Part model, mm, in its own coordinate system. A direction names the side the tool comes from. Give positions to 0.01 mm unless a question says otherwise; leave off trailing zeros. Write each loop counter-clockwise with the first axis right and the second up, starting at its lowest first coordinate (ties: lowest second). Pieces come first, ordered by that corner, then holes. Notation, with made-up numbers: M -24.5,31 L 3.5,31 A17 cw 3.5,58 Z; hole C 11,60.25 d4. An arc over 180 degrees is marked long. Answer as CSV lines item,"result". Start each with the question number.
1) Slice it at A-A, the plane y = 0. Give the cut face in (x, z), plus the area to 3 significant figures.
2) Slice it at C-C, the plane y = 7. Give the cut face in (x, z).
3) Slice it at D-D, the plane x = 5.25. Give the cut face in (y, z).
4) Tool access for faces 1 (the cylindrical face through (-3, 0, 1)), 2 (the cylindrical face through (0, -6, 1)), 3 (the cylindrical face through (-1.08, -4.88, 3.99)): list every direction of +Z, -Z, +X, -X, +Y, -Y with a clear straight run to the whole face (end or side of a thin tool).
5) Mould opens along Y. For faces 4 (the cylindrical face through (-5.95, 4.99, 1.48)), 5 (the flat face through (-1.2, 1.2, 5)), 6 (the cylindrical face through (-2.17, -9.76, 1.48)) say: pulls with the +Y half, pulls with the -Y half, needs draft (parallel to the pull), parting line crosses it, or undercut.
6) Wall check: line 1 along Y through (x, z) = (0, 2.4); line 2 along Y through (x, z) = (0, 4.25); line 3 along Z through (x, y) = (7.75, 3). Give the ranges that are in metal, low to high. Write a range as from..to.
7) Pin check, flat tips, straight feed: pin 1 Ø1.5 at (x, z) = (-1.5, 4) entering from +Y; pin 2 Ø2.5 at (x, y) = (4.95, 4.95) entering from +Z; pin 3 Ø1.8 at (x, y) = (-0.5, -0.5) entering from -Z. Stop position of each tip, or through.
```python
from build123d import *

# Parameters (mm, degrees)
SKETCH_1_R      = 10
SKETCH_1_R_2    = 3
SKETCH_1_R_3    = 1
EXTRUDE_1_DEPTH = 3
SKETCH_2_R      = 5
SKETCH_2_R_2    = 1.5
EXTRUDE_2_DEPTH = 2


with BuildPart() as part:
    # 草图1 → 凸台-拉伸1 (new body)
    with BuildSketch(Plane.XY):
        Circle(SKETCH_1_R)
        Circle(SKETCH_1_R_2, mode=Mode.SUBTRACT)
        with Locations((7, 0)):
            Circle(SKETCH_1_R_3, mode=Mode.SUBTRACT)
        with Locations((4.949747468, -4.949747468)):
            Circle(SKETCH_1_R_3, mode=Mode.SUBTRACT)
        with Locations((0, -7)):
            Circle(SKETCH_1_R_3, mode=Mode.SUBTRACT)
        with Locations((-4.949747468, -4.949747468)):
            Circle(SKETCH_1_R_3, mode=Mode.SUBTRACT)
        with Locations((-7, 0)):
            Circle(SKETCH_1_R_3, mode=Mode.SUBTRACT)
        with Locations((-4.949747468, 4.949747468)):
            Circle(SKETCH_1_R_3, mode=Mode.SUBTRACT)
        with Locations((0, 7)):
            Circle(SKETCH_1_R_3, mode=Mode.SUBTRACT)
        with Locations((4.949747468, 4.949747468)):
            Circle(SKETCH_1_R_3, mode=Mode.SUBTRACT)
    extrude(amount=EXTRUDE_1_DEPTH)

    # 草图2 → 凸台-拉伸2 (add)
    with BuildSketch(Plane.XY.offset(3)):
        Circle(SKETCH_2_R)
        Circle(SKETCH_2_R_2, mode=Mode.SUBTRACT)
    extrude(amount=EXTRUDE_2_DEPTH)


solid = part.part
```
Found:
1,outline,"M -10,0 L -8,0 L -8,3 L -10,3 Z; M -6,0 L -3,0 L -3,3 L -1.5,3 L -1.5,5 L -5,5 L -5,3 L -6,3 Z; M 1.5,3 L 3,3 L 3,0 L 6,0 L 6,3 L 5,3 L 5,5 L 1.5,5 Z; M 8,0 L 10,0 L 10,3 L 8,3 Z"
1,area,"44.0 mm²"
2,outline,"M -7.14,0 L -1,0 L -1,3 L -7.14,3 Z; M 1,0 L 7.14,0 L 7.14,3 L 1,3 Z"
3,outline,"M -8.51,0 L -5.9,0 L -5.9,3 L -8.51,3 Z; M -4,0 L 4,0 L 4,3 L -4,3 Z; M 5.9,0 L 8.51,0 L 8.51,3 L 5.9,3 Z"
4,face 1,"-Z"
4,face 2,"+Z, -Z"
4,face 3,"+Z"
5,face 4,"undercut"
5,face 5,"needs draft"
5,face 6,"parting line crosses it"
6,line 1,"-10..-8, -6..-3, 3..6, 8..10"
6,line 2,"-5..-1.5, 1.5..5"
6,line 3,"0..3"
7,pin 1,"y = 4.94"
7,pin 2,"z = 3"
7,pin 3,"z = 3"
